Verification items for the finished model (mm, model axes). Face numbers are marked on the shaded views. A direction names the side the tool comes from. Give positions to 0.01 mm unless a question says otherwise; leave off trailing zeros. Order: outer loops, then holes, each group sorted by start corner. A loop starts at its lowest first (then second) coordinate and runs counter-clockwise, first axis right, second up. Notation, with made-up numbers: (4.5, 20.25) -> (11.5, 20.25) arc R19 ccw to (11.5, 48.25) -> close; hole circle Ø9 at (-21, -22.5). An arc over 180 degrees is marked (long way). One line per question, with ' | ' between items. Start each with the question number.
Q1. Section check A-A on x = 0. Record the cut outline in (y, z) (3 decimals).
Q2. Material ranges on probe 1 along Y at (x, z) = (-25, -10); probe 2 along Y at (x, z) = (-6, 7) (3 decimals); probe 3 along Z at (x, y) = (1.5, 13.5) (3 decimals), recorded low to high. Write a range as [from, to].
Q3. Section check D-D on z = -4.25. Record the cut outline in (x, y) (3 decimals), plus the area to 3 significant figures.
Q4. Section check B-B on x = -15.5. Record the cut outline in (y, z) (3 decimals), plus the area to 3 significant figures.
Q5. Access from +Z, -Z, +X, -X, +Y, -Y to the whole of each face (thin tool, end or side, straight path). Record for the marked faces 1 and 2.
Q6. Section check C-C on y = 8. Record the cut outline in (x, z) (3 decimals), plus the area to 3 significant figures.
Q7. Go/stop test with a flat-tipped pin: pin 1 (6.5 mm diameter, centred on x = -2, z = -1.5, fed in from +Y) (3 decimals). Record where the tip stops, or that it passes through.
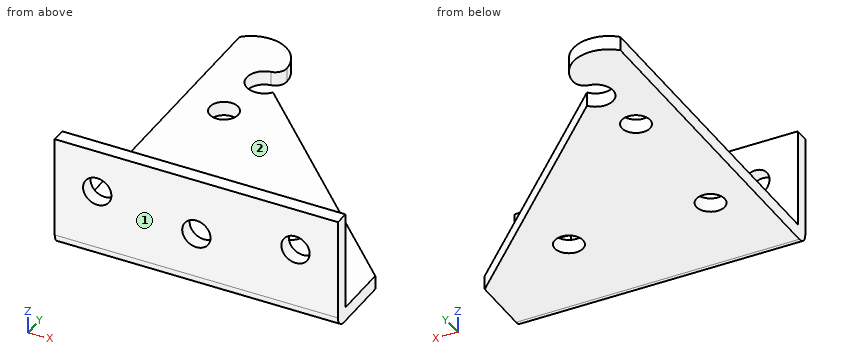
from build123d import *

# Parameters (mm, degrees)
SKETCH1_W           = 63.5
SKETCH1_H           = 25.4
SKETCH1_R           = 3.175
BOSS_EXTRUDE1_DEPTH = 3.175
SKETCH2_R           = 3.175
BOSS_EXTRUDE2_DEPTH = 3.175
FILLET2_R           = 2.54


with BuildPart() as part:
    # Sketch1 → Boss-Extrude1 (new body)
    with BuildSketch(Plane(origin=(0, 0, 0), x_dir=(1, 0, 0), z_dir=(0, 1, 0))):
        Rectangle(SKETCH1_W, SKETCH1_H)
        with Locations(Location((-22.225, -3.175, 0), (0, 0, 270))):
            Circle(SKETCH1_R, mode=Mode.SUBTRACT)
        with Locations(Location((0, 0, 0), (0, 0, 270))):
            Circle(SKETCH1_R, mode=Mode.SUBTRACT)
        with Locations(Location((22.225, -3.175, 0), (0, 0, 90))):
            Circle(SKETCH1_R, mode=Mode.SUBTRACT)
    extrude(amount=BOSS_EXTRUDE1_DEPTH)

    # Sketch2 → Boss-Extrude2 (add)
    with BuildSketch(Plane.XY.offset(-12.7)):
        with BuildLine():
            Line((-31.75, 0), (-31.75, 78.705067014))
            ThreePointArc((-31.75, 78.705067014), (-23.163673383, 80.377738088), (-18.238159017, 73.148482141))
            ThreePointArc((-18.238159017, 73.148482141), (-18.843460583, 71.462906002), (-20.410488317, 70.595737627))
            ThreePointArc((-20.410488317, 70.595737627), (-23.244591892, 64.65221549), (-16.669658329, 64.294658329))
            Line((-16.669658329, 64.294658329), (31.75, 15.875))
            Line((31.75, 15.875), (31.75, 0))
            Line((31.75, 0), (-31.75, 0))
        make_face()
        with Locations((-22.225, 53.975)):
            Circle(SKETCH2_R, mode=Mode.SUBTRACT)
        with Locations((-22.225, 22.225)):
            Circle(SKETCH2_R, mode=Mode.SUBTRACT)
        with Locations((9.525, 22.225)):
            Circle(SKETCH2_R, mode=Mode.SUBTRACT)
    extrude(amount=BOSS_EXTRUDE2_DEPTH)

    # Fillet2
    fillet2_edges = [part.edges().sort_by_distance(p)[0] for p in [
        (0, 0, -12.7),
    ]]
    fillet(fillet2_edges, radius=FILLET2_R)


solid = part.part
Filled in:
1) outline: (0, -10.16) arc R2.54 ccw to (2.54, -12.7) -> (47.625, -12.7) -> (47.625, -9.525) -> (3.175, -9.525) -> (3.175, -3.175) -> (0, -3.175) -> close; (0, 3.175) -> (3.175, 3.175) -> (3.175, 12.7) -> (0, 12.7) -> close
2) probe 1: [0, 20.68], [23.77, 52.43], [55.52, 80.89] | probe 2: [0, 3.175] | probe 3: [-12.7, -9.525]
3) outline: (-31.75, 0) -> (31.75, 0) -> (31.75, 3.175) -> (-31.75, 3.175) -> close | area: 202 mm²
4) outline: (0, -10.16) arc R2.54 ccw to (2.54, -12.7) -> (63.125, -12.7) -> (63.125, -9.525) -> (3.175, -9.525) -> (3.175, 12.7) -> (0, 12.7) -> close | area: 270 mm²
5) face 1: +Z, -Z, +X, -X, -Y | face 2: +Z, +X, -X, +Y
6) outline: (-31.75, -12.7) -> (31.75, -12.7) -> (31.75, -9.525) -> (-31.75, -9.525) -> close | area: 202 mm²
7) pin 1: y = 3.175
